from build123d import *

# Parameters (mm, degrees)
LPATTERN1_COUNT = 2
LPATTERN1_PITCH = 3.4


with BuildPart() as part:
    # Sketch1 → Revolve1 (revolve)
    with BuildSketch(Plane.XY, mode=Mode.PRIVATE) as revolve1_sk:
        Polygon((0, 4), (0, 5), (20, 5), (20, 0), (-200, 0), (-200, 4), align=None)
    revolve(revolve1_sk.sketch.rotate(Axis((-200, 0, 0), (1, 0, 0)), 90), axis=Axis((-200, 0, 0), (1, 0, 0)))

    # Sketch2 → Revolve2 (revolve)
    with BuildSketch(Plane.XY, mode=Mode.PRIVATE) as revolve2_sk:
        Polygon((15.405, -125), (15.405, -115), (15.58, -115), (15.58, -95), (16.08, -95), (16.08, 0), (15.03, 0), (15.03, -125), align=None)
    revolve2 = revolve(revolve2_sk.sketch.rotate(Axis((15.03, 0, 0), (0, -1, 0)), 180), axis=Axis((15.03, 0, 0), (0, -1, 0)))

    # LPattern1: Revolve2 ×2
    with Locations(*[(-i * LPATTERN1_PITCH, 0, 0) for i in range(1, LPATTERN1_COUNT)]):
        add(revolve2)

    # Sketch3 → Revolve3 (revolve)
    with BuildSketch(Plane.XY, mode=Mode.PRIVATE) as revolve3_sk:
        Polygon((15.03, -13), (16.08, -13), (16.23, -13.850692273), (16.23, -27.149307727), (16.08, -28), (15.03, -28), align=None)
    revolve(revolve3_sk.sketch.rotate(Axis((15.03, -13, 0), (0, -1, 0)), 180), axis=Axis((15.03, -13, 0), (0, -1, 0)))

    # Sketch4 → Revolve4 (revolve)
    with BuildSketch(Plane.XY, mode=Mode.PRIVATE) as revolve4_sk:
        Polygon((11.63, -20.5), (12.68, -20.5), (12.83, -21.350692273), (12.83, -34.649307727), (12.68, -35.5), (11.63, -35.5), align=None)
    revolve(revolve4_sk.sketch.rotate(Axis((11.63, -20.5, 0), (0, -1, 0)), 180), axis=Axis((11.63, -20.5, 0), (0, -1, 0)))


solid = part.part
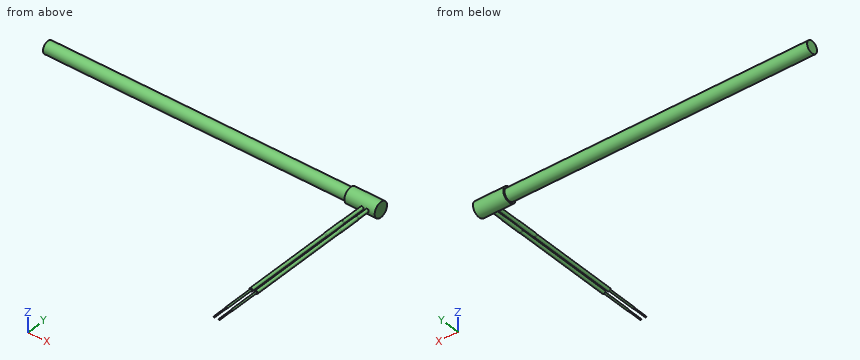
Verification items for the finished model (mm, model axes). Coordinates: 2 decimals unless noted, no trailing zeros. Order: outer loops, then holes, each group sorted by start corner. A loop starts at its lowest first (then second) coordinate and runs counter-clockwise, first axis right, second up. Notation, with made-up numbers: M 11,25.5 L 70,25.5 A9 ccw 70,39.5 Z; hole C 46,2 d11. An arc over 180 degrees is marked long. One line per item, written item: value. Start each with the question number.
Item 1: Sectioned sample at A-A on y = 0. Record the cut outline in (x, z), then the cut area to 3 significant figures.
Item 2: Thickness scan on probe 1 along X at (y, z) = (-71, -0.25); probe 2 along Z at (x, y) = (-128.5, -0.5); probe 3 along X at (y, z) = (-53.5, -0.5). Record the ranges inside material, lowest first.
Item 3: Sectioned sample at C-C on x = -169.5. Record the cut outline in (y, z).
Item 4: Sectioned sample at B-B on y = -74. Record the cut outline in (x, z), then the cut area to 3 significant figures.
Item 5: Sectioned sample at D-D on y = -23.5. Record the cut outline in (x, z).
Item 6: Depth check by flat-ended pin: P1, Ø1, axis at y = -23.5, z = 3, coming from the +X side. Enter the tip coordinate at first touch or a pass-through.
Calculated:
1. outline: M -200,-4 L 0,-4 L 0,-5 L 20,-5 L 20,5 L 0,5 L 0,4 L -200,4 Z
1. area: 1,800 mm^2
2. probe 1: 10.61 to 12.65, 14.01 to 16.05
2. probe 2: -3.97 to 3.97
2. probe 3: 10.71 to 12.55, 14.11 to 15.95
3. outline: C 0,0 d8
4. outline: C 11.63,0 d2.1; C 15.03,0 d2.1
4. area: 6.93 mm^2
5. outline: C 11.63,0 d2.4; C 15.03,0 d2.4
6. P1: through
